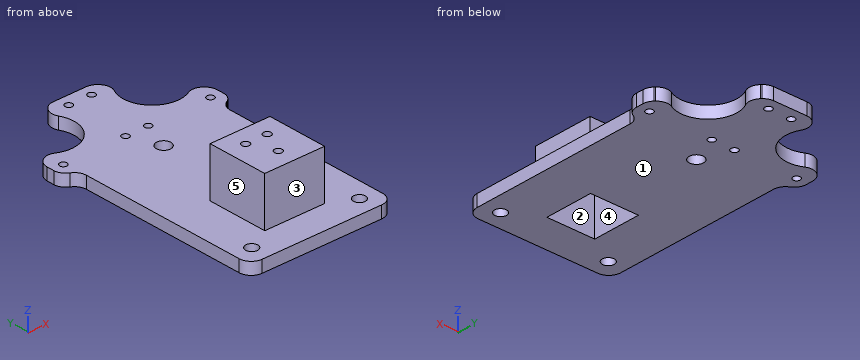
from build123d import *

# Parameters (mm, degrees)
F0_R     = 2.5
F0_R_2   = 1.5
F0_R_3   = 3
F1_DEPTH = 5
F2_R     = 5
F3_R     = 5
F4_W     = 25
F4_H     = 25
F5_DEPTH = 20.4
F6_W     = 20
F6_H     = 20
F7_DEPTH = 22.9
F8_R     = 1.6
F9_DEPTH = 25.4010001


with BuildPart() as f1:
    # F0 (on Top) → F1 (new body)
    with BuildSketch(Plane.XY):
        with BuildLine():
            Line((0, 80), (0, 0))
            Line((0, 0), (60, 0))
            Line((60, 0), (60, 80))
            Line((60, 80), (65.5, 80))
            Line((65.5, 80), (65.5, 89))
            Line((65.5, 89), (60.7352813742, 93.7647186258))
            ThreePointArc((60.7352813742, 93.7647186258), (43.7647186258, 93.7647186258), (43.7647186258, 110.7352813742))
            Line((43.7647186258, 110.7352813742), (39, 115.5))
            Line((39, 115.5), (21, 115.5))
            Line((21, 115.5), (16.2352813742, 110.7352813742))
            ThreePointArc((16.2352813742, 110.7352813742), (16.2352813742, 93.7647186258), (-0.7352813742, 93.7647186258))
            Line((-0.7352813742, 93.7647186258), (-5.5, 89))
            Line((-5.5, 89), (-5.5, 80))
            Line((-5.5, 80), (0, 80))
        make_face()
        with Locations((7.5, 7.5)):
            Circle(F0_R, mode=Mode.SUBTRACT)
        with Locations((52.5, 7.5)):
            Circle(F0_R, mode=Mode.SUBTRACT)
        with Locations((-0.75, 84.75)):
            Circle(F0_R_2, mode=Mode.SUBTRACT)
        with Locations((25.25, 84.75)):
            Circle(F0_R_2, mode=Mode.SUBTRACT)
        with Locations((25.25, 110.75)):
            Circle(F0_R_2, mode=Mode.SUBTRACT)
        with Locations((30, 72.5)):
            Circle(F0_R_3, mode=Mode.SUBTRACT)
        with Locations((34.75, 84.75)):
            Circle(F0_R_2, mode=Mode.SUBTRACT)
        with Locations((60.75, 84.75)):
            Circle(F0_R_2, mode=Mode.SUBTRACT)
        with Locations((34.75, 110.75)):
            Circle(F0_R_2, mode=Mode.SUBTRACT)
    extrude(amount=F1_DEPTH)

    # F2
    f2_edges = [f1.edges().sort_by_distance(p)[0] for p in [
        (0, 0, 2.5),
        (60, 0, 2.5),
        (-0.735281, 93.764719, 2.5),
        (-5.5, 89, 2.5),
        (0, 80, 2.5),
        (60, 80, 2.5),
        (65.5, 89, 2.5),
        (60.735281, 93.764719, 2.5),
        (43.764719, 110.735281, 2.5),
        (39, 115.5, 2.5),
        (21, 115.5, 2.5),
        (16.235281, 110.735281, 2.5),
    ]]
    fillet(f2_edges, radius=F2_R)

    # F3
    f3_edges = [f1.edges().sort_by_distance(p)[0] for p in [
        (-5.5, 80, 2.5),
        (65.5, 80, 2.5),
    ]]
    fillet(f3_edges, radius=F3_R)

    # F4 (on face) → F5 (join)
    with BuildSketch(Plane.XY.offset(5)):
        with Locations((30, 25)):
            Rectangle(F4_W, F4_H)
    extrude(amount=F5_DEPTH)

    # F6 (on face) → F7 (cut)
    with BuildSketch(Plane(origin=(0, 0, 0), x_dir=(1, 0, 0), z_dir=(0, 0, -1))):
        with Locations((30, -25)):
            Rectangle(F6_W, F6_H)
    extrude(amount=-F7_DEPTH, mode=Mode.SUBTRACT)

    # F8 (on face) → F9 (cut, through all)
    with BuildSketch(Plane.XY.offset(25.4)):
        with Locations((25.5, 30)):
            Circle(F8_R)
        with Locations((30, 20)):
            Circle(F8_R)
        with Locations((34.5, 30)):
            Circle(F8_R)
    extrude(amount=-F9_DEPTH, mode=Mode.SUBTRACT)


solid = f1.part
For this review, take the finished solid that the model builds, in its own axes (mm). Face numbers are marked on the shaded views. A direction names the side the tool comes from. Round coordinates to 2 decimals unless told otherwise and drop trailing zeros. Loops run counter-clockwise (first coordinate to the right, second up) from the corner with the lowest first, then second, coordinate; pieces in that order, holes last. Notation, with made-up numbers: (55.5, -14) - (89.5, -14) arc R17 cw to (89.5, -5) - close; hole circle Ø5 at (-13.5, -20). An arc over 180 degrees is marked (long way). One line per item, written item: value. Start each with the question number.
Item 1: Take a section at B-B (y = 72.5). Give the boundary of the cut face in (x, z).
Item 2: The part is to be moulded in two halves that separate along Y. For the marked faces 3, 4 and 5, say which applies: +Y half, -Y half, draft (parallel to the pull), parting line (faces both ways), or undercut.
Item 3: Take a section at A-A (z = 12.25). Give the boundary of the cut face in (x, y), plus the area to 3 significant figures.
Item 4: For L1, parallel to Y at x = 30, z = 3; L2, parallel to X at y = 84.75, z = 4.05; L3, parallel to Y at x = 34.75, z = 2.35, list the stretches that pass through material, from the lowest coordinate up.
Item 5: Take a section at C-C (x = 30). Give the boundary of the cut face in (y, z).
Item 6: Take a section at D-D (y = 7.5). Give the boundary of the cut face in (x, z), plus the area to 3 significant figures.
Item 7: For the marked faces 1 and 2, list the 3-axis set-ups (+Z, -Z, +X, -X, +Y, -Y) from which the entire face can be reached by the end or side of a thin tool; tool diameter is ignored.
Item 8: Clearance check with flat-ended pins moving along their axes: pin 1 Ø10 at (x, z) = (34, 12) entering from -Y; pin 2 Ø8 at (x, y) = (32.5, 47.5) entering from +Z; pin 3 Ø2.5 at (y, z) = (45.5, 2) entering from +X. State where each tip first meets the part, or that it passes through.
Answer below:
1. outline: (0, 0) - (27, 0) - (27, 5) - (0, 5) - close; (33, 0) - (60, 0) - (60, 5) - (33, 5) - close
2. face 3: -Y half
2. face 4: undercut
2. face 5: draft
3. outline: (17.5, 12.5) - (42.5, 12.5) - (42.5, 37.5) - (17.5, 37.5) - close; hole (20, 15) - (40, 15) - (40, 35) - (20, 35) - close
3. area: 225 mm2
4. L1: y = 0 to 15, 35 to 69.5, 75.5 to 115.5
4. L2: x = -5.5 to -2.25, 0.75 to 23.75, 26.75 to 33.25, 36.25 to 59.25, 62.25 to 65.5
4. L3: y = 0 to 15, 35 to 83.25, 86.25 to 109.25, 112.25 to 115.5
5. outline: (0, 0) - (15, 0) - (15, 22.9) - (18.4, 22.9) - (18.4, 25.4) - (12.5, 25.4) - (12.5, 5) - (0, 5) - close; (21.6, 22.9) - (35, 22.9) - (35, 0) - (69.5, 0) - (69.5, 5) - (37.5, 5) - (37.5, 25.4) - (21.6, 25.4) - close; (75.5, 0) - (115.5, 0) - (115.5, 5) - (75.5, 5) - close
6. outline: (0, 0) - (5, 0) - (5, 5) - (0, 5) - close; (10, 0) - (50, 0) - (50, 5) - (10, 5) - close; (55, 0) - (60, 0) - (60, 5) - (55, 5) - close
6. area: 250 mm2
7. face 1: -Z, +X, -X, +Y, -Y
7. face 2: -Z
8. pin 1: stops at y = 12.5
8. pin 2: stops at z = 5
8. pin 3: stops at x = 60
